Part model, mm, in its own coordinate system. Face numbers are marked on the shaded views. A direction names the side the tool comes from. Coordinates: 2 decimals unless noted, no trailing zeros. Order: outer loops, then holes, each group sorted by start corner. A loop starts at its lowest first (then second) coordinate and runs counter-clockwise, first axis right, second up. Notation, with made-up numbers: M -25,-21.5 L -16,-21.5 A16 ccw -16,-9.5 Z; hole C 3,33 d6. An arc over 180 degrees is marked long. Answer in a Markdown table with one row per item. Add a question column.
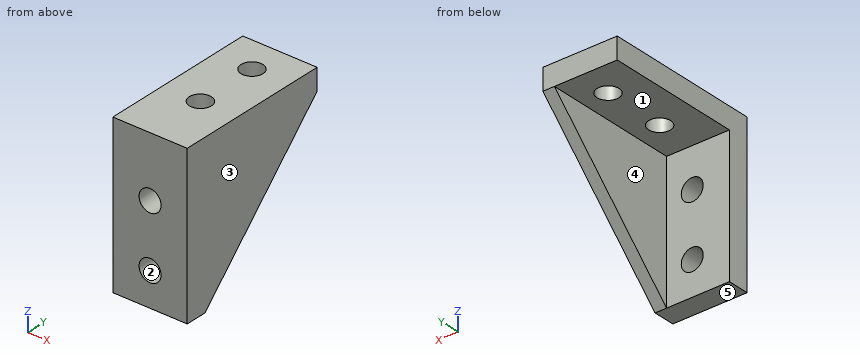
Autodesk Inventor part; units mm, degrees
ref_plane "YZ Plane" through (0, 0, 0) normal (1, 0, 0) x (0, 1, 0)
ref_plane "XZ Plane" through (0, 0, 0) normal (0, 1, 0) x (-1, 0, 0)
ref_plane "XY Plane" through (0, 0, 0) normal (0, 0, 1) x (1, 0, 0)
sketch "Sketch1" plane through (0, 0, 0) normal (1, 0, 0) x (0, 1, 0)
  line L0 (0, 0) -> (0, -37.75)
  line L1 (0, -37.75) -> (5.15, -37.75)
  line L2 (5.15, -37.75) -> (37.75, -5.15)
  line L3 (37.75, -5.15) -> (37.75, 0)
  line L4 (37.75, 0) -> (0, 0)
  dimension "d0" = 135
  dimension "d1" = 37.75
  dimension "d2" = 5.15
  dimension "d3" = 5.15
extrude "Extrusion1" add sketch "Sketch1" against normal blind 2.75
sketch "Sketch2" plane through (-2.75, 0, 0) normal (-1, 0, 0) x (0, 0, 1)
  line L0 (-37.75, 5.15) -> (-37.75, 0)
  line L1 (-37.75, 0) -> (0, 0)
  line L2 (0, 0) -> (0, 37.75)
  line L3 (0, 37.75) -> (-5.15, 37.75)
  line L4 (-5.15, 37.75) -> (-37.75, 5.15)
  line L5 (-37.75, 5.15) -> (-37.75, 0)
  line L6 (-37.75, 5.15) -> (-5.15, 5.15)
  line L7 (0, 37.75) -> (-5.15, 37.75)
  line L8 (-5.15, 5.15) -> (-5.15, 37.75)
extrude "Extrusion2" add sketch "Sketch2" along normal blind 15 contours L6 L8 L3 L2 L1 L0
sketch "Sketch3" plane through (-2.75, 5.15, -5.15) normal (0, 1, 0) x (1, 0, 0)
  line L0 (0, 0) -> (-15, 0) construction
  line L1 (-6.125, 0.4254) -> (-6.125, 32.6) construction
  line L2 (2.75, 32.6) -> (-15, 32.6) construction
  circle A0 centre (-6.125, 24.475) radius 2.625
  circle A1 centre (-6.125, 9.475) radius 2.625
  line L3 (-6.125, 2.1875) -> (-15, 2.1875) construction
  line L4 (-15, 32.6) -> (-15, -5.15) construction
  line L5 (-6.125, 2.1875) -> (2.75, 2.1875) construction
  line L6 (2.75, -5.15) -> (2.75, 32.6) construction
  dimension "d8" = 5.25
  dimension "d9" = 8.125
  dimension "d10" = 5.25
  dimension "d11" = 23.125
extrude "Extrusion3" cut sketch "Sketch3" against normal up to next
sketch "Sketch4" plane through (-2.75, 5.15, -5.15) normal (0, 0, -1) x (-1, 0, 0)
  line L0 (0, 0) -> (15, 0) construction
  line L1 (6.125, -0.1704) -> (6.125, 32.4296) construction
  line L2 (0, 32.6) -> (15, 32.6) construction
  circle A0 centre (6.125, 24.475) radius 2.625
  circle A1 centre (6.125, 9.475) radius 2.625
  line L3 (6.125, 29.763) -> (15, 29.763) construction
  line L4 (15, 32.6) -> (15, 0) construction
  line L5 (6.125, 29.763) -> (-2.75, 29.763) construction
  line L6 (-2.75, 32.6) -> (-2.75, -5.15) construction
  dimension "d14" = 5.25
  dimension "d15" = 5.25
  dimension "d16" = 8.125
  dimension "d17" = 23.125
extrude "Extrusion4" cut sketch "Sketch4" against normal up to next
equation "\"d3\" = d2"
equation "\"d10\" = d8"
equation "\"d15\" = d14"
properties part number "2020 Extrusion 90deg 4Hole Aluminum Bracket"
(1) 3-axis set-ups, long thin cutter, end or side, ignore diameter. For the marked faces 4 and 5: which of +Z, -Z, +X, -X, +Y, -Y reach the whole face in a straight line?
(2) Slice it at C-C (y = 24). List the corners of the cut face in (x, z), and give its area (3 significant figures).
(3) Slice it at D-D (z = -14). List the corners of the cut face in (x, y).
(4) Slice it at B-B (z = -33.5). List the corners of the cut face in (x, y).
(5) Pull direction Z, two halves, no side cores. Call the marked faces 1, 2 and 3: pulls with the +Z half, pulls with the -Z half, needs draft (parallel to the pull), parting line crosses it, or undercut.
(6) Wall check: line 1 (Y direction, x = -8.5, z = -3); line 2 (Y direction, x = -15, z = -12); line 3 (X direction, y = 16, z = -9). Give the ranges that are in metal, low to high.
(7) Drop flat-ended pins along their axis: P1, Ø3, axis at x = -8.875, y = 29.625, coming from the +Z side; P2, Ø7.5, axis at x = -9, z = -24, coming from the +Y side; P3, Ø16.5, axis at y = 16.5, z = -17.5, coming from the -X side; P4, Ø6, axis at x = -2.5, y = 33.5, coming from the -Z side. Give the stop position or say it passes through.
(8) Slice it at A-A (x = -8). List the corners of the cut face in (y, z).
Computed:
| question | item | result |
|---|---|---|
| 1 | face 4 | -Z, -X, +Y |
| 1 | face 5 | -Z, +X, -X, +Y, -Y |
| 2 | outline | M -17.75,-5.15 L -2.75,-5.15 L -2.75,-18.9 L 0,-18.9 L 0,0 L -17.75,0 Z |
| 2 | area | 129 mm^2 |
| 3 | outline | M -17.75,0 L -11.42,0 L -11.42,5.15 L -17.75,5.15 Z; M -6.33,0 L 0,0 L 0,28.9 L -2.75,28.9 L -2.75,5.15 L -6.33,5.15 Z |
| 4 | outline | M -17.75,0 L 0,0 L 0,9.4 L -2.75,9.4 L -2.75,5.15 L -17.75,5.15 Z |
| 5 | face 1 | pulls with the -Z half |
| 5 | face 2 | undercut |
| 5 | face 3 | needs draft |
| 6 | line 1 | y = 0 to 12.03, 17.22 to 27.03, 32.22 to 37.75 |
| 6 | line 2 | y = 0 to 5.15 |
| 6 | line 3 | x = -2.75 to 0 |
| 7 | P1 | passes through |
| 7 | P2 | stops at y = 5.15 |
| 7 | P3 | stops at x = -2.75 |
| 7 | P4 | stops at z = -12.4 |
| 8 | outline | M 0,-37.75 L 5.15,-37.75 L 5.15,-32.1 L 0,-32.1 Z; M 0,-27.15 L 5.15,-27.15 L 5.15,-17.1 L 0,-17.1 Z; M 0,-12.15 L 5.15,-12.15 L 5.15,-5.15 L 12.15,-5.15 L 12.15,0 L 0,0 Z; M 17.1,-5.15 L 27.15,-5.15 L 27.15,0 L 17.1,0 Z; M 32.1,-5.15 L 37.75,-5.15 L 37.75,0 L 32.1,0 Z |
